Check sheet for the drawn part. Datum: minimum x, y, z corner. Units: mm. A direction names the side the tool comes from. Round coordinates to 2 decimals unless told otherwise and drop trailing zeros. Order: outer loops, then holes, each group sorted by start corner. A loop starts at its lowest first (then second) coordinate and runs counter-clockwise, first axis right, second up.
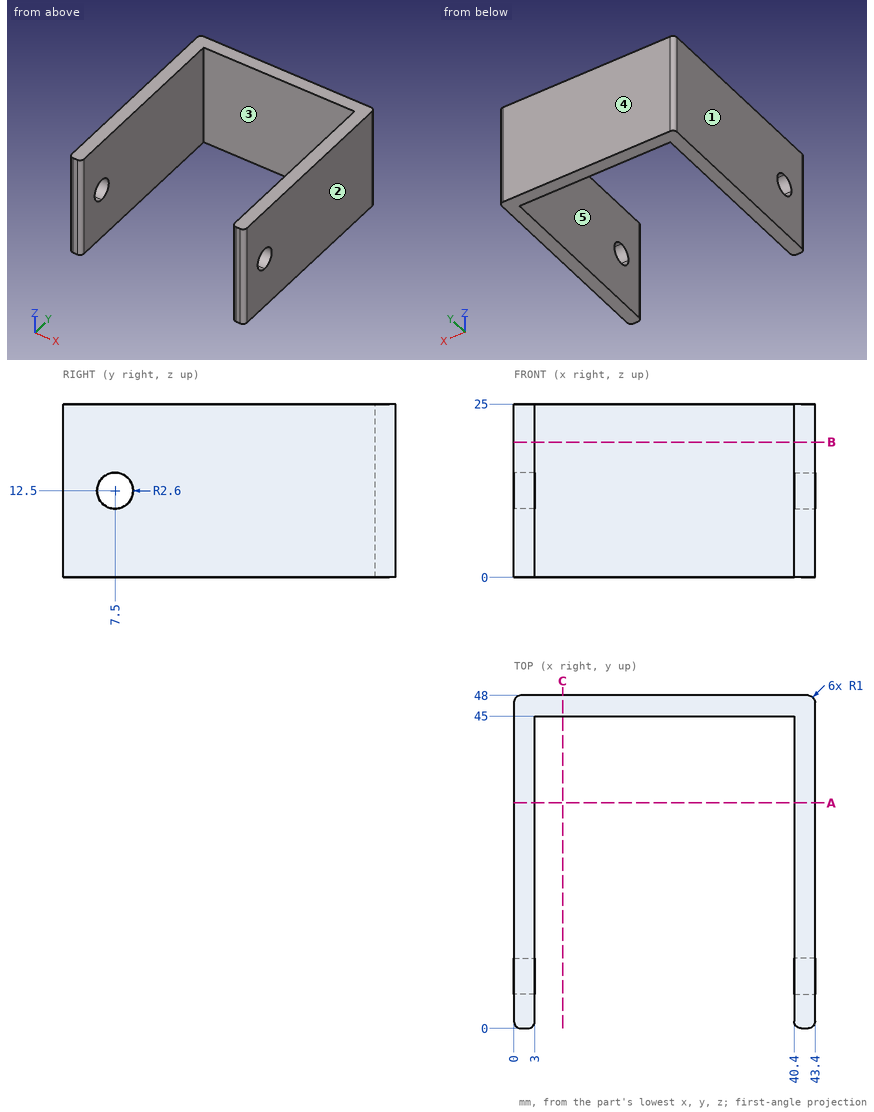
(1) Draft check along X on the marked faces 1, 2 and 3. Enter one of: released by +X, released by -X, zero draft, split by the parting line, or undercut.
Returned:
face 1: released by -X
face 2: released by +X
face 3: undercut
(2) Set-up check for the marked faces 4 and 5: record each of +Z, -Z, +X, -X, +Y, -Y from which the full face is reachable in a straight line by a thin tool's end or side.
Returned:
face 4: +Z, -Z, +X, -X, +Y
face 5: +Z, -Z, -Y
(3) Sectioned sample at B-B, the plane z = 19.5. Record the cut outline in (x, y).
Returned:
outline: (0, 1) arc R1 ccw to (1, 0) - (2, 0) arc R1 ccw to (3, 1) - (3, 45) - (40.4, 45) - (40.4, 1) arc R1 ccw to (41.4, 0) - (42.4, 0) arc R1 ccw to (43.4, 1) - (43.4, 47) arc R1 ccw to (42.4, 48) - (1, 48) arc R1 ccw to (0, 47) - close
(4) Sectioned sample at A-A, the plane y = 32.5. Record the cut outline in (x, z).
Returned:
outline: (0, 0) - (3, 0) - (3, 25) - (0, 25) - close; (40.4, 0) - (43.4, 0) - (43.4, 25) - (40.4, 25) - close
(5) Material ranges on line 1 (X direction, y = 12, z = 13.75); line 2 (Y direction, x = 38, z = 13.5); line 3 (Z direction, x = 2, y = 9), recorded low to high.
Returned:
line 1: x = 0 to 3, 40.4 to 43.4
line 2: y = 45 to 48
line 3: z = 0 to 10.38, 14.62 to 25
(6) Depth check by flat-ended pin: P1, Ø8, axis at x = 29, z = 9, coming from the -Y side. Enter the tip coordinate at first touch or a pass-through.
Returned:
P1: stops at y = 45
(7) Sectioned sample at C-C, the plane x = 7. Record the cut outline in (y, z).
Returned:
outline: (45, 0) - (48, 0) - (48, 25) - (45, 25) - close
